Autodesk Inventor part; units mm, degrees
ref_plane "YZ Plane" through (0, 0, 0) normal (1, 0, 0) x (0, 1, 0)
ref_plane "XZ Plane" through (0, 0, 0) normal (0, 1, 0) x (-1, 0, 0)
ref_plane "XY Plane" through (0, 0, 0) normal (0, 0, 1) x (1, 0, 0)
sketch "Sketch1" plane through (0, 0, 0) normal (0, 1, 0) x (-1, 0, 0)
  line L0 (0, -5.6886) -> (6.7556, -12.4442)
  line L1 (6.7556, -12.4442) -> (5.3414, -13.8584)
  line L2 (9.5, -18.017) -> (5.3414, -13.8584)
  line L3 (10, -18.017) -> (9.5, -18.017)
  line L4 (10, -18.017) -> (10, 0)
  line L5 (0, 0) -> (10, 0)
  line L6 (0, 0) -> (0, -5.6886)
  circle A0 centre (5, -2.8443) radius 1.339
extrude "Extrusion1" add sketch "Sketch1" along normal blind 10
sketch "Sketch2" plane through (0, 10, 0) normal (0, 1, 0) x (1, 0, 0)
  line L0 (0, 5.6886) -> (-10, 5.6886)
  line L1 (-10, 5.6886) -> (-10, 0)
  line L2 (-10, 0) -> (0, 0)
  line L3 (0, 0) -> (0, 5.6886)
extrude "Extrusion2" add sketch "Sketch2" along normal blind 20
sketch "Sketch3" plane through (0, 0, 0) normal (0, -1, 0) x (1, 0, 0)
  circle A0 centre (-5, -2.8443) radius 1.339
hole "Hole1" at (-5, 0, -2.8443) direction (0, 1, 0) diameter 4.318 end through all
sketch "Sketch8" plane through (-9.5, 0, -18.017) normal (0.7071068, 0, -0.7071068) x (-0.7071068, 0, -0.7071068)
  line L0 (-5.8811, 0) -> (0, 0)
  line L1 (0, 0) -> (0, 10)
  line L2 (-5.8811, 10) -> (0, 10)
  line L3 (-5.8811, 0) -> (-5.8811, 10)
  line L4 (-1.0406, 1) -> (-4.8406, 1)
  line L5 (-4.8406, 1) -> (-4.8406, 9)
  line L6 (-4.8406, 9) -> (-1.0406, 9)
  line L7 (-1.0406, 9) -> (-1.0406, 1)
  line L8 (-1.0406, 1) -> (-4.8406, 9) construction
  line L9 (-4.8406, 1) -> (-1.0406, 9) construction
  point P0 (-19.4575, 0)
  point P1 (-2.9406, 5)
  dimension "d41" = 3.8
  dimension "d42" = 8
extrude "Extrusion6" add sketch "Sketch8" along normal blind 2.5
sketch "Sketch9" plane through (-6.0772, 1, -14.5942) normal (-0.7071068, 0, -0.7071068) x (-0.7071068, 0, 0.7071068)
  line L0 (-2.25, 7) -> (-1.75, 7)
  line L1 (-1.75, 7) -> (-1.75, 6.5)
  line L2 (-1.75, 6.5) -> (-2.25, 6.5)
  line L3 (-2.25, 6.5) -> (-2.25, 7)
  line L4 (-1.75, 1) -> (-2.25, 1)
  line L5 (-2.25, 1) -> (-2.25, 1.5)
  line L6 (-2.25, 1.5) -> (-1.75, 1.5)
  line L7 (-1.75, 1.5) -> (-1.75, 1)
  point P0 (6.0224, -1)
  dimension "d45" = 0.5
  dimension "d46" = 0.5
  dimension "d47" = 0.5
  dimension "d48" = 0.5
extrude "Extrusion7" add sketch "Sketch9" along normal blind 4
sketch "Sketch10" plane through (0, 30, 0) normal (0, 1, 0) x (1, 0, 0)
  circle A0 centre (-5, 2.8443) radius 2.159
  line L0 (0, 5.6886) -> (-10, 5.6886)
  line L1 (-10, 5.6886) -> (-10, 0)
  line L2 (-10, 0) -> (0, 0)
  line L3 (0, 0) -> (0, 5.6886)
extrude "Extrusion8" cut sketch "Sketch10" against normal blind 15
sketch "Sketch11" plane through (-10, 0, -18.017) normal (-1, 0, 0) x (0, 0, 1)
  line L0 (18.017, 15) -> (12.3284, 15)
  line L1 (12.3284, 10) -> (12.3284, 15)
  line L2 (0, 10) -> (12.3284, 10)
  line L3 (0, 0) -> (0, 10)
  line L4 (0, 0) -> (18.017, 0)
  line L5 (18.017, 0) -> (18.017, 15)
extrude "Extrusion9" cut sketch "Sketch11" against normal blind 0.5
properties part number "TensionMountV2"
The listing builds one solid part. Answer for the finished solid, in the listing's coordinates (mm). A direction names the side the tool comes from. Round coordinates to 2 decimals unless told otherwise and drop trailing zeros. Loops run counter-clockwise (first coordinate to the right, second up) from the corner with the lowest first, then second, coordinate; pieces in that order, holes last. Notation, with made-up numbers: (-39, -39.5) - (0, -39.5) arc R17 cw to (0, -32.5) - close; hole circle Ø6 at (-20.75, 78.5). An arc over 180 degrees is marked (long way). Return JSON: item names as keys, results as strings. Group by question number.
1. The part is cut by section C-C on y = 11. Determine the outline of the cut face in (x, z), then the cut area to 3 significant figures.
2. The part is cut by section B-B on z = -2.5. Determine the outline of the cut face in (x, y).
3. Each of these flat-tipped pins is pushed along its axis until it touches: P1, Ø2.5, axis at x = -6.5, z = -17.5, coming from the +Y side; P2, Ø2.5, axis at x = -5, y = 12.5, coming from the -Z side; P3, Ø1, axis at x = -6, y = 8, coming from the -Z side; P4, Ø3.5, axis at x = -5, z = -2.84, coming from the +Y side. Where does it stop, or does it pass through?
4. Which of the six approach directions +Z, -Z, +X, -X, +Y, -Y give full straight-line access (tool end or side, diameter ignored) to faces 1 (the flat face through (-6.164, 7.754, -17.156)), 2 (the cylindrical face through (-3.085, 7.605, -3.841)), 3 (the flat face through (-3, 15, -4)), 4 (the flat face through (-3.33, 4.93, -9.02))?
5. The part is cut by section A-A on x = -3.25. Determine the outline of the cut face in (y, z), then the cut area to 3 significant figures.
6. The mould has two halves that part along Z. Classify faces 5 (the flat face through (-7.893, 5.056, -18.153)), 6 (the flat face through (-7, 10, -11)), 7 (the flat face through (-5, 12, -5.689)), 8 (the flat face through (-5, 7, 0)): pulls with the +Z half, pulls with the -Z half, needs draft (parallel to the pull), parting line crosses it, or undercut.
7. The part is cut by section D-D on z = -9. Determine the outline of the cut face in (x, y).
8. Consider probe 1 along Z at (x, y) = (-5, 12); probe 2 along Z at (x, y) = (-5.25, 4.75); probe 3 along Z at (x, y) = (-5, 9.75). Determine where each line is inside the solid, lowest interval first.
Resolved:
{
 "1": {"outline": "(-9.5, -5.69) - (0, -5.69) - (0, 0) - (-9.5, 0) - close; hole circle Ø4.32 at (-5, -2.84)", "area": "39.4 mm²"},
 "2": {"outline": "(-9.5, 0) - (-7.13, 0) - (-7.13, 15) - (-9.5, 15) - close; (-2.87, 0) - (0, 0) - (0, 15) - (-2.87, 15) - close"},
 "3": {"P1": "stops at y = 10", "P2": "stops at z = -5.69", "P3": "stops at z = -18.2", "P4": "passes through"},
 "4": {"face 1": "none", "face 2": "+Y, -Y", "face 3": "+Z, -Z, +X, -X, +Y", "face 4": "+X, +Y, -Y"},
 "5": {"outline": "(0, -8.94) - (10, -8.94) - (10, -5.69) - (15, -5.69) - (15, -4.11) - (0, -4.11) - close; (0, -1.58) - (15, -1.58) - (15, 0) - (0, 0) - close", "area": "79.9 mm²"},
 "6": {"face 5": "undercut", "face 6": "needs draft", "face 7": "pulls with the -Z half", "face 8": "pulls with the +Z half"},
 "7": {"outline": "(-9.5, 0) - (-3.31, 0) - (-3.31, 10) - (-9.5, 10) - close"},
 "8": {"probe 1": "z = -5.69 to -5, -0.69 to 0", "probe 2": "z = -15.42 to -13.95, -10.94 to -4.99, -0.7 to 0", "probe 3": "z = -17.05 to -14.2, -10.69 to -5, -0.69 to 0"}
}
